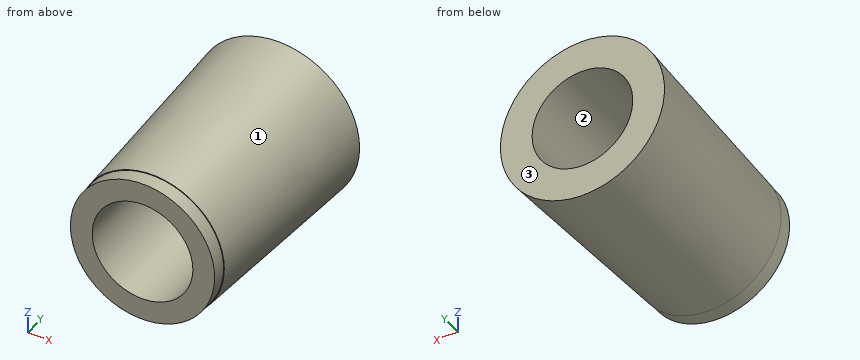
from build123d import *

# Parameters (mm, degrees)
F0_R      = 5.5
F2_DEPTH  = 14
F1_R      = 4.835
F3_DEPTH  = 15
F3_FACE_R = 4.835
F2_FACE_R = 5.5
F5_R      = 3.375
F6_DEPTH  = 16


with BuildPart() as f2:
    # F0 (on Front) → F2 (new body)
    with BuildSketch(Plane.XZ):
        Circle(F0_R)
    extrude(amount=F2_DEPTH)

    # F1 (on Front) → F3 (join)
    with BuildSketch(Plane.XZ):
        Circle(F1_R)
    extrude(amount=F3_DEPTH)

    # F3_face (on face) → F4 section 0
    with BuildSketch(Plane.XZ.offset(15)):
        Circle(F3_FACE_R)
    # F2_face (on face) → F4 section 1
    with BuildSketch(Plane(origin=(0, 0, 0), x_dir=(1, 0, 0), z_dir=(0, 1, 0))):
        Circle(F2_FACE_R)
    loft(mode=Mode.INTERSECT)

    # F5 (on face) → F6 (cut)
    with BuildSketch(Plane.XZ.offset(15)):
        Circle(F5_R)
    extrude(amount=-F6_DEPTH, mode=Mode.SUBTRACT)


solid = f2.part
Check sheet for the modelled part. Datum: model origin and axes. Units: mm. Face numbers are marked on the shaded views. Round coordinates to 2 decimals unless told otherwise and drop trailing zeros. Loops run counter-clockwise (first coordinate to the right, second up) from the corner with the lowest first, then second, coordinate; pieces in that order, holes last. Notation, with made-up numbers: (22.5, 85.5) -> (49.5, 85.5) arc R29 cw to (49.5, 110.5) -> close; hole circle Ø11 at (64, 21.25). An arc over 180 degrees is marked (long way). Put each result on its own line as item: value. Start each with the question number.
1. Draft check along Z on the marked faces 1, 2 and 3. Enter one of: +Z half, -Z half, draft (parallel to the pull), parting line (faces both ways), or undercut.
2. Gauge pin test, flat ends, axial feed: pin 1 (1.5 mm diameter, centred on x = 2, z = -1.5, fed in from +Y); pin 2 (6 mm diameter, centred on x = 1.5, y = -6, fed in from -Z); pin 3 (1.5 mm diameter, centred on y = -7, z = -2.5, fed in from -X); pin 4 (4 mm diameter, centred on x = 3.5, y = -9.5, fed in from -Z). Record the tip position at first contact, or that the pin passes through.
3. Section check A-A (x = 0). Enter the section's corners in (y, z) (3 decimals), plus the area to 3 significant figures.
4. Scan lines: probe 1 along Z at (x, y) = (0, -7) (3 decimals); probe 2 along Z at (x, y) = (-1, -4.75); probe 3 along X at (y, z) = (-13.5, 1.25). Record each from-to range of solid material in increasing order.
Findings:
1. face 1: parting line
1. face 2: undercut
1. face 3: draft
2. pin 1: passes through
2. pin 2: stops at z = -5.35
2. pin 3: stops at x = -4.89
2. pin 4: stops at z = -4.86
3. outline: (-15, -4.835) -> (-14, -4.835) -> (-14, -4.879) -> (0, -5.5) -> (0, -3.375) -> (-15, -3.375) -> close; (-15, 3.375) -> (0, 3.375) -> (0, 5.5) -> (-14, 4.879) -> (-14, 4.835) -> (-15, 4.835) -> close
3. area: 53.7 mm^2
4. probe 1: z = -5.19 to -3.375, 3.375 to 5.19
4. probe 2: z = -5.19 to -3.22, 3.22 to 5.19
4. probe 3: x = -4.74 to -3.13, 3.13 to 4.74
